```python
from build123d import *

# Parameters (mm, degrees)
ESQUISSE1_W      = 60
ESQUISSE1_H      = 40
ESQUISSE1_R      = 2.5
ESQUISSE1_R_2    = 2
EXTRUSION1_DEPTH = 8
ESQUISSE2_R      = 4
EXTRUSION2_DEPTH = 4
ESQUISSE3_R      = 2
EXTRUSION3_DEPTH = 15
ESQUISSE4_W      = 10
ESQUISSE4_H      = 5
EXTRUSION4_DEPTH = 41


with BuildPart() as part:
    # Esquisse1 → Extrusion1 (new body)
    with BuildSketch(Plane.XY):
        Rectangle(ESQUISSE1_W, ESQUISSE1_H)
        Circle(ESQUISSE1_R, mode=Mode.SUBTRACT)
        with Locations((9.899494937, 9.899494937)):
            Circle(ESQUISSE1_R_2, mode=Mode.SUBTRACT)
        with Locations((0, 14)):
            Circle(ESQUISSE1_R_2, mode=Mode.SUBTRACT)
        with Locations((14, 0)):
            Circle(ESQUISSE1_R_2, mode=Mode.SUBTRACT)
        with Locations((9.899494937, -9.899494937)):
            Circle(ESQUISSE1_R_2, mode=Mode.SUBTRACT)
        with Locations((0, -14)):
            Circle(ESQUISSE1_R_2, mode=Mode.SUBTRACT)
        with Locations((-9.899494937, -9.899494937)):
            Circle(ESQUISSE1_R_2, mode=Mode.SUBTRACT)
        with Locations((-14, 0)):
            Circle(ESQUISSE1_R_2, mode=Mode.SUBTRACT)
        with Locations((-9.899494937, 9.899494937)):
            Circle(ESQUISSE1_R_2, mode=Mode.SUBTRACT)
    extrude(amount=EXTRUSION1_DEPTH)

    # Esquisse2 → Extrusion2 (cut)
    with BuildSketch(Plane.XY):
        Circle(ESQUISSE2_R)
    extrude(amount=EXTRUSION2_DEPTH, mode=Mode.SUBTRACT)

    # Esquisse3 → Extrusion3 (cut)
    with BuildSketch(Plane.XZ.offset(20)):
        with Locations((-15.5, 4)):
            Circle(ESQUISSE3_R)
        with Locations((15.5, 4)):
            Circle(ESQUISSE3_R)
    extrude(amount=-EXTRUSION3_DEPTH, mode=Mode.SUBTRACT)

    # Esquisse4 → Extrusion4 (cut, through all)
    with BuildSketch(Plane(origin=(0, 20, 0), x_dir=(1, 0, 0), z_dir=(0, 1, 0))):
        with Locations((-23, -5.5)):
            Rectangle(ESQUISSE4_W, ESQUISSE4_H)
        with Locations((23, -5.5)):
            Rectangle(ESQUISSE4_W, ESQUISSE4_H)
    extrude(amount=-EXTRUSION4_DEPTH, mode=Mode.SUBTRACT)


solid = part.part
```
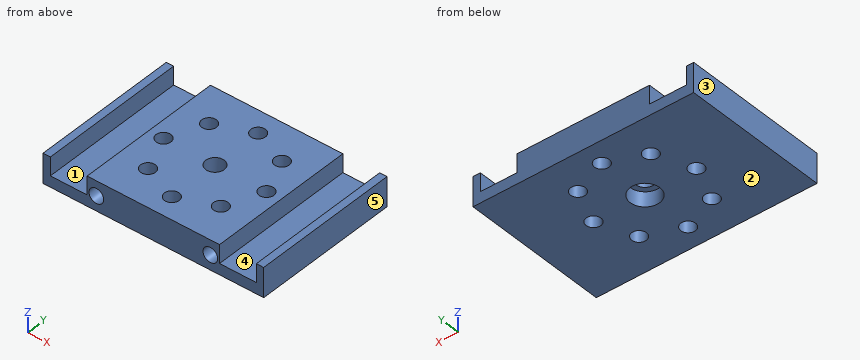
Here's how the part is built. I have some questions about the finished solid (model axes, mm). Face numbers are marked on the shaded views. A direction names the side the tool comes from. Round coordinates to 2 decimals unless told otherwise and drop trailing zeros. Order: outer loops, then holes, each group sorted by start corner. A loop starts at its lowest first (then second) coordinate and runs counter-clockwise, first axis right, second up. Notation, with made-up numbers: (44.25, -37.75) -> (64.25, -37.75) arc R21 ccw to (64.25, -4.75) -> close; hole circle Ø7 at (50, 1). An arc over 180 degrees is marked (long way). Use a Markdown table: item, result. Add a question column.
(1) If we mould it in two halves opening along X, with no side actions, what happens to the marked faces 3, 4 and 5? For each: released by +X, released by -X, zero draft, split by the parting line, or undercut.
(2) For pin 1 Ø3 at (x, y) = (-22, 9) entering from +Z; pin 2 Ø4.5 at (x, y) = (-9.9, -9.9) entering from -Z; pin 3 Ø3 at (x, y) = (-9.9, 9.9) entering from -Z; pin 4 Ø3 at (x, z) = (-15.5, 4) entering from -Y, each with a flat end and sliding along its axis, tell me the tip position at first contact or that it passes through.
(3) Suppose I cut it at C-C, the plane x = 11. Please give me the cut outline in (y, z).
(4) Suppose I cut it at B-B, the plane x = 0. Please give me the cut outline in (y, z), and give its area (3 significant figures).
(5) Suppose I cut it at A-A, the plane y = 14. Please give me the cut outline in (x, z), and give its area (3 significant figures).
(6) Suppose I cut it at D-D, the plane y = 0. Please give me the cut outline in (x, z), and give its area (3 significant figures).
(7) For the marked faces 1 and 2, which set-ups out of +Z, -Z, +X, -X, +Y, -Y let a thin tool reach every point of the face, with its end or its side?
(8) I need wall thicknesses on line 1 along Y through (x, z) = (0, 5.5); line 2 along X through (y, z) = (-10, 7); line 3 along X through (y, z) = (-10, 1.5). Which ranges of each line are inside material? Lowest first, please.
Verdict:
| question | item | result |
|---|---|---|
| 1 | face 3 | released by -X |
| 1 | face 4 | undercut |
| 1 | face 5 | released by +X |
| 2 | pin 1 | z = 3 |
| 2 | pin 2 | z = 0 |
| 2 | pin 3 | through |
| 2 | pin 4 | y = -5 |
| 3 | outline | (-20, 0) -> (-11.57, 0) -> (-11.57, 8) -> (-20, 8) -> close; (-8.23, 0) -> (8.23, 0) -> (8.23, 8) -> (-8.23, 8) -> close; (11.57, 0) -> (20, 0) -> (20, 8) -> (11.57, 8) -> close |
| 4 | outline | (-20, 0) -> (-16, 0) -> (-16, 8) -> (-20, 8) -> close; (-12, 0) -> (-4, 0) -> (-4, 4) -> (-2.5, 4) -> (-2.5, 8) -> (-12, 8) -> close; (2.5, 4) -> (4, 4) -> (4, 0) -> (12, 0) -> (12, 8) -> (2.5, 8) -> close; (16, 0) -> (20, 0) -> (20, 8) -> (16, 8) -> close |
| 4 | area | 204 mm2 |
| 5 | outline | (-30, 0) -> (-2, 0) -> (-2, 8) -> (-18, 8) -> (-18, 3) -> (-28, 3) -> (-28, 8) -> (-30, 8) -> close; (2, 0) -> (30, 0) -> (30, 8) -> (28, 8) -> (28, 3) -> (18, 3) -> (18, 8) -> (2, 8) -> close |
| 5 | area | 348 mm2 |
| 6 | outline | (-30, 0) -> (-16, 0) -> (-16, 8) -> (-18, 8) -> (-18, 3) -> (-28, 3) -> (-28, 8) -> (-30, 8) -> close; (-12, 0) -> (-4, 0) -> (-4, 4) -> (-2.5, 4) -> (-2.5, 8) -> (-12, 8) -> close; (2.5, 4) -> (4, 4) -> (4, 0) -> (12, 0) -> (12, 8) -> (2.5, 8) -> close; (16, 0) -> (30, 0) -> (30, 8) -> (28, 8) -> (28, 3) -> (18, 3) -> (18, 8) -> (16, 8) -> close |
| 6 | area | 264 mm2 |
| 7 | face 1 | +Z, +Y, -Y |
| 7 | face 2 | -Z, +X, -X, +Y, -Y |
| 8 | line 1 | -20 to -16, -12 to -2.5, 2.5 to 12, 16 to 20 |
| 8 | line 2 | -30 to -28, -18 to -11.9, -7.9 to 7.9, 11.9 to 18, 28 to 30 |
| 8 | line 3 | -30 to -11.9, -7.9 to 7.9, 11.9 to 30 |
